```python
from build123d import *

# Parameters (mm, degrees)
F0_R     = 7
F1_DEPTH = 12
F2_W     = 85
F2_H     = 25
F3_DEPTH = 25
F5_DEPTH = 3


with BuildPart() as f1:
    # F0 (on Front) → F1 (new body)
    with BuildSketch(Plane.XZ):
        with BuildLine():
            Line((285, 0), (0, 0))
            Line((0, 0), (-365, 0))
            Line((-365, 0), (-365, -75))
            ThreePointArc((-365, -75), (-357.67767, -92.67767), (-340, -100))
            Line((-340, -100), (-48.660254, -100))
            ThreePointArc((-48.660254, -100), (-42.189778, -99.148146), (-36.160254, -96.650635))
            Line((-36.160254, -96.650635), (47.5, -48.349365))
            ThreePointArc((47.5, -48.349365), (53.529524, -45.851854), (60, -45))
            Line((60, -45), (280, -45))
            ThreePointArc((280, -45), (283.535534, -43.535534), (285, -40))
            Line((285, -40), (285, 0))
        make_face()
        with Locations((40, -17.5)):
            Circle(F0_R, mode=Mode.SUBTRACT)
        with Locations((260, -17.5)):
            Circle(F0_R, mode=Mode.SUBTRACT)
    extrude(amount=F1_DEPTH)

    # F2 (on face) → F3 (cut)
    with BuildSketch(Plane(origin=(0, 0, 0), x_dir=(-1, 0, 0), z_dir=(0, 1, 0))):
        with Locations((39.5, -37.5)):
            Rectangle(F2_W, F2_H)
    extrude(amount=-F3_DEPTH, mode=Mode.SUBTRACT)

    # F4 (on face) → F5 (join)
    with BuildSketch(Plane.YZ.offset(285)):
        with BuildLine():
            Line((-12, -40), (-6, -40))
            Line((-6, -40), (0, -40))
            Line((0, -40), (66.827433, -6.887593))
            ThreePointArc((66.827433, -6.887593), (76.970455, 2.331662), (80.727967, 15.513341))
            Line((80.727967, 15.513341), (80.727967, 138.932179))
            ThreePointArc((80.727967, 138.932179), (73.405636, 156.609848), (55.727967, 163.932179))
            Line((55.727967, 163.932179), (0, 163.932179))
            Line((0, 163.932179), (-12, 163.932179))
            Line((-12, 163.932179), (-67.727967, 163.932179))
            ThreePointArc((-67.727967, 163.932179), (-85.405636, 156.609848), (-92.727967, 138.932179))
            Line((-92.727967, 138.932179), (-92.727967, 15.513341))
            ThreePointArc((-92.727967, 15.513341), (-88.970455, 2.331662), (-78.827433, -6.887593))
            Line((-78.827433, -6.887593), (-12, -40))
        make_face()
    extrude(amount=F5_DEPTH)


solid = f1.part
```
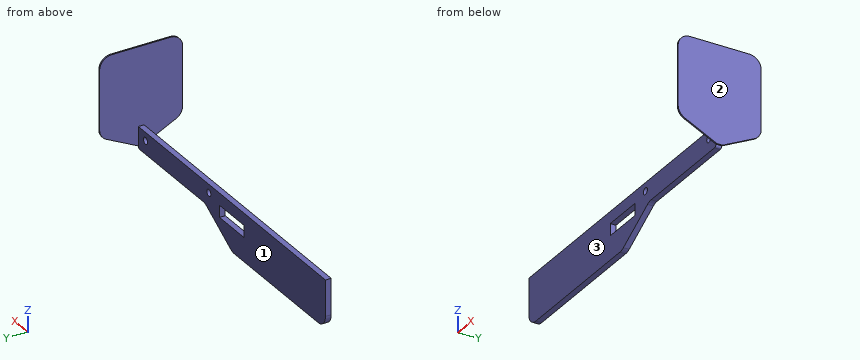
Design review of the part built by this model. Coordinates are the model's own, in mm. Face numbers are marked on the shaded views. A direction names the side the tool comes from. Coordinates: 2 decimals unless noted, no trailing zeros. Write each loop counter-clockwise with the first axis right and the second up, starting at its lowest first coordinate (ties: lowest second). Pieces come first, ordered by that corner, then holes.
1) Add section C-C (x = 40). Write out the cut boundary in (y, z).
2) Add section A-A (x = 260). Write out the cut boundary in (y, z), plus the area to 3 significant figures.
3) To check wall thickness, follow L1, parallel to X at y = -9, z = -17; L2, parallel to X at y = 4, z = 70.5; L3, parallel to Z at x = 260, y = -3. State the ranges of each line that lie inside material, in increasing order.
4) Machinability: for the marked faces 1, 2 and 3, which of the approach directions +Z, -Z, +X, -X, +Y, -Y give a long, thin tool a straight path to every point of the face, cutting with its end or side? Answer none if there is none.
5) Add section D-D (z = 39). Write out the cut boundary in (x, y).
6) Add section B-B (z = -17.5). Write out the cut boundary in (x, y), plus the area to 3 significant figures.
7) Insertion check: pin 1 (10 mm diameter, centred on x = -283, z = -54.5, fed in from +Y); pin 2 (9.5 mm diameter, centred on x = -31.5, y = -7, fed in from +Z); pin 3 (16 mm diameter, centred on x = 260, z = -17.5, fed in from -Y). Each pin has a flat end and moves straight along its axis. Give the tip position at first contact, or say it passes through.
Check result:
1. outline: (-12, -52.68) - (0, -52.68) - (0, -24.5) - (-12, -24.5) - close; (-12, -10.5) - (0, -10.5) - (0, 0) - (-12, 0) - close
2. outline: (-12, -45) - (0, -45) - (0, -24.5) - (-12, -24.5) - close; (-12, -10.5) - (0, -10.5) - (0, 0) - (-12, 0) - close
2. area: 372 mm2
3. L1: x = -365 to 33.02, 46.98 to 253.02, 266.98 to 288
3. L2: x = 285 to 288
3. L3: z = -45 to -24.5, -10.5 to 0
4. face 1: +Z, -Z, -X, +Y
4. face 2: +Z, -Z, +X, +Y, -Y
4. face 3: +Z, -Z, -X, -Y
5. outline: (285, -92.73) - (288, -92.73) - (288, 80.73) - (285, 80.73) - close
6. outline: (-365, -12) - (33, -12) - (33, 0) - (-365, 0) - close; (47, -12) - (253, -12) - (253, 0) - (47, 0) - close; (267, -12) - (285, -12) - (285, -57.41) - (288, -57.41) - (288, 45.41) - (285, 45.41) - (285, 0) - (267, 0) - close
6. area: 7,770 mm2
7. pin 1: stops at y = 0
7. pin 2: stops at z = 0
7. pin 3: stops at y = -12
